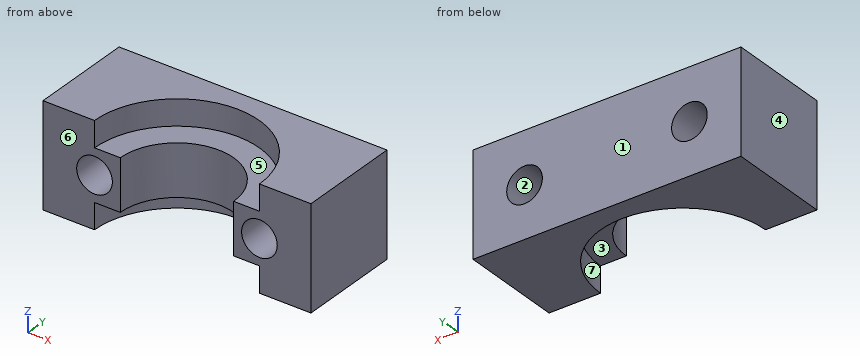
from build123d import *

# Parameters (mm, degrees)
RESSALTO_EXTRUS_O1_DEPTH = 2.5
RESSALTO_EXTRUS_O2_DEPTH = 5
ESBO_O2_R                = 1.730913938
CORTE_EXTRUS_O1_DEPTH    = 15


with BuildPart() as part:
    # Esboço1 → Ressalto-extrusão1 (new, symmetric)
    with BuildSketch(Plane.XY):
        with BuildLine():
            Line((-5.5, 0), (-13, 0))
            Line((-13, 0), (-13, 10))
            Line((-13, 10), (13, 10))
            Line((13, 10), (13, 0))
            Line((13, 0), (5.5, 0))
            ThreePointArc((5.5, 0), (0, 5.5), (-5.5, 0))
        make_face()
    extrude(amount=RESSALTO_EXTRUS_O1_DEPTH, both=True)

    # Esboço3 → Ressalto-extrusão2 (add, symmetric)
    with BuildSketch(Plane.XY):
        with BuildLine():
            Line((-13, 10), (-13, 0))
            Line((-13, 0), (-8, 0))
            ThreePointArc((-8, 0), (0, 8), (8, 0))
            Line((8, 0), (13, 0))
            Line((13, 0), (13, 10))
            Line((13, 10), (-13, 10))
        make_face()
    extrude(amount=RESSALTO_EXTRUS_O2_DEPTH, both=True)

    # Esboço2 → Corte-extrusão1 (cut)
    with BuildSketch(Plane.XZ):
        with Locations((-8, 0)):
            Circle(ESBO_O2_R)
        with Locations((8, 0)):
            Circle(ESBO_O2_R)
    extrude(amount=-CORTE_EXTRUS_O1_DEPTH, mode=Mode.SUBTRACT)


solid = part.part
Geometry check sheet. Reference: the model listing, model coordinates, mm. Face numbers are marked on the shaded views. A direction names the side the tool comes from. Round coordinates to 2 decimals unless told otherwise and drop trailing zeros. Write each loop counter-clockwise with the first axis right and the second up, starting at its lowest first coordinate (ties: lowest second). Pieces come first, ordered by that corner, then holes. Notation, with made-up numbers: (78, 81.25) -> (93, 81.25) arc R35 ccw to (93, 113.25) -> close; hole circle Ø2 at (60, 8.5). An arc over 180 degrees is marked (long way). One line per item, written item: value. Start each with the question number.
(1) Cross-section at C-C, the plane x = -7. Record the cut outline in (y, z), and give its area (3 significant figures).
(2) Cross-section at D-D, the plane y = 6.5. Record the cut outline in (x, z), and give its area (3 significant figures).
(3) Draft check along X on the marked faces 1, 2, 3 and 4. Enter one of: +X half, -X half, draft (parallel to the pull), parting line (faces both ways), or undercut.
(4) Cross-section at B-B, the plane z = 0. Record the cut outline in (x, y).
(5) Go/stop test with a flat-tipped pin: pin 1 Ø3 at (x, z) = (-3, 0.5) entering from -Y. Record where the tip stops, or that it passes through.
(6) Scan lines: line 1 (Z direction, x = 8, y = 2); line 2 (X direction, y = 1, z = -0.75); line 3 (X direction, y = 0.5, z = -1.5). Record each from-to range of solid material in increasing order. Write a range as [from, to].
(7) Access from +Z, -Z, +X, -X, +Y, -Y to the whole of each face (thin tool, end or side, straight path). Record for the marked faces 5, 6 and 7.
(8) Cross-section at A-A, the plane y = 4.75. Record the cut outline in (x, z), and give its area (3 significant figures).
Answer:
1. outline: (0, -2.5) -> (3.87, -2.5) -> (3.87, -5) -> (10, -5) -> (10, -1.41) -> (0, -1.41) -> close; (0, 1.41) -> (10, 1.41) -> (10, 5) -> (3.87, 5) -> (3.87, 2.5) -> (0, 2.5) -> close
1. area: 52.4 mm²
2. outline: (-13, -5) -> (-4.66, -5) -> (-4.66, -2.5) -> (4.66, -2.5) -> (4.66, -5) -> (13, -5) -> (13, 5) -> (4.66, 5) -> (4.66, 2.5) -> (-4.66, 2.5) -> (-4.66, 5) -> (-13, 5) -> close; hole circle Ø3.46 at (-8, 0); hole circle Ø3.46 at (8, 0)
2. area: 195 mm²
3. face 1: draft
3. face 2: undercut
3. face 3: undercut
3. face 4: -X half
4. outline: (-13, 0) -> (-9.73, 0) -> (-9.73, 10) -> (-13, 10) -> close; (-6.27, 0) -> (-5.5, 0) arc R5.5 cw to (5.5, 0) -> (6.27, 0) -> (6.27, 10) -> (-6.27, 10) -> close; (9.73, 0) -> (13, 0) -> (13, 10) -> (9.73, 10) -> close
5. pin 1: y = 3.16
6. line 1: [-5, -1.73], [1.73, 5]
6. line 2: [-13, -9.56], [-6.44, -5.41], [5.41, 6.44], [9.56, 13]
6. line 3: [-13, -8.86], [-7.14, -5.48], [5.48, 7.14], [8.86, 13]
7. face 5: +Z, -Y
7. face 6: +Z, -Z, +X, -X, -Y
7. face 7: -Z, -Y
8. outline: (-13, -5) -> (-6.44, -5) -> (-6.44, -2.5) -> (-2.77, -2.5) -> (-2.77, 2.5) -> (-6.44, 2.5) -> (-6.44, 5) -> (-13, 5) -> close; (2.77, -2.5) -> (6.44, -2.5) -> (6.44, -5) -> (13, -5) -> (13, 5) -> (6.44, 5) -> (6.44, 2.5) -> (2.77, 2.5) -> close; hole circle Ø3.46 at (-8, 0); hole circle Ø3.46 at (8, 0)
8. area: 149 mm²
